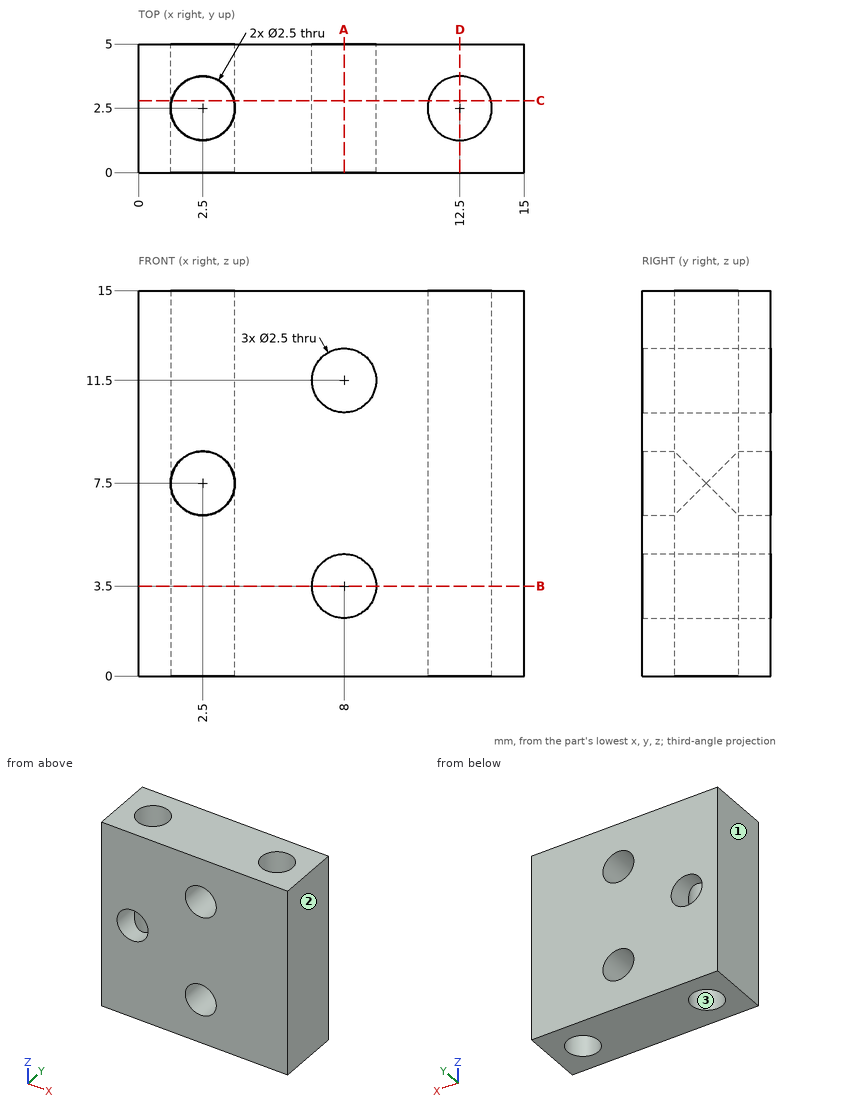
The drawing under review shows one solid part. Ordinate dimensions are in mm from its lowest x, y, z. Round coordinates to 2 decimals unless told otherwise and drop trailing zeros. Order: outer loops, then holes, each group sorted by start corner. A loop starts at its lowest first (then second) coordinate and runs counter-clockwise, first axis right, second up. Notation, with made-up numbers: (69.25, 16.5) -> (111.25, 16.5) arc R11 cw to (111.25, 27.5) -> close; hole circle Ø6 at (-19, 28.25). An arc over 180 degrees is marked (long way). Use a Markdown table: item, result.
Item 1: Take a section at B-B (z = 3.5). State the section outline as (x, y) points, plus the area to 3 significant figures.
Resolved:
| item | result |
|---|---|
| outline | (0, 0) -> (6.75, 0) -> (6.75, 5) -> (0, 5) -> close; (9.25, 0) -> (15, 0) -> (15, 5) -> (9.25, 5) -> close; hole circle Ø2.5 at (2.5, 2.5); hole circle Ø2.5 at (12.5, 2.5) |
| area | 52.7 mm² |
Item 2: Take a section at D-D (x = 12.5). State the section outline as (y, z) points.
Resolved:
| item | result |
|---|---|
| outline | (0, 0) -> (1.25, 0) -> (1.25, 15) -> (0, 15) -> close; (3.75, 0) -> (5, 0) -> (5, 15) -> (3.75, 15) -> close |
Item 3: Take a section at A-A (x = 8). State the section outline as (y, z) points, plus the area to 3 significant figures.
Resolved:
| item | result |
|---|---|
| outline | (0, 0) -> (5, 0) -> (5, 2.25) -> (0, 2.25) -> close; (0, 4.75) -> (5, 4.75) -> (5, 10.25) -> (0, 10.25) -> close; (0, 12.75) -> (5, 12.75) -> (5, 15) -> (0, 15) -> close |
| area | 50.0 mm² |
Item 4: Draft analysis for pull direction X (two halves, no side actions). For the marked faces 1, 2 and 3, state which applies: +X half, -X half, draft (parallel to the pull), parting line (faces both ways), or undercut.
Resolved:
| item | result |
|---|---|
| face 1 | -X half |
| face 2 | +X half |
| face 3 | undercut |
Item 5: For pin 1 (1.5 mm diameter, centred on x = 8, z = 3.5, fed in from +Y), flat-tipped, find the tip position at first contact; note if it passes through.
Resolved:
| item | result |
|---|---|
| pin 1 | passes through |
Item 6: Take a section at C-C (y = 2.8). State the section outline as (x, z) points, plus the area to 3 significant figures.
Resolved:
| item | result |
|---|---|
| outline | (0, 0) -> (1.29, 0) -> (1.29, 7.2) arc R1.25 cw to (1.29, 7.8) -> (1.29, 15) -> (0, 15) -> close; (3.71, 0) -> (11.29, 0) -> (11.29, 15) -> (3.71, 15) -> (3.71, 7.8) arc R1.25 cw to (3.71, 7.2) -> close; (13.71, 0) -> (15, 0) -> (15, 15) -> (13.71, 15) -> close; hole circle Ø2.5 at (8, 3.5); hole circle Ø2.5 at (8, 11.5) |
| area | 142 mm² |
Item 7: For line 1 along Z through (x, y) = (8, 2.5); line 2 along Z through (x, y) = (2.5, 4.35); line 3 along X through (y, z) = (3.25, 10.5), list the stretches that pass through material, from the lowest coordinate up. Write a range as [from, to].
Resolved:
| item | result |
|---|---|
| line 1 | z = [0, 2.25], [4.75, 10.25], [12.75, 15] |
| line 2 | z = [0, 6.25], [8.75, 15] |
| line 3 | x = [0, 1.5], [3.5, 7.25], [8.75, 11.5], [13.5, 15] |
